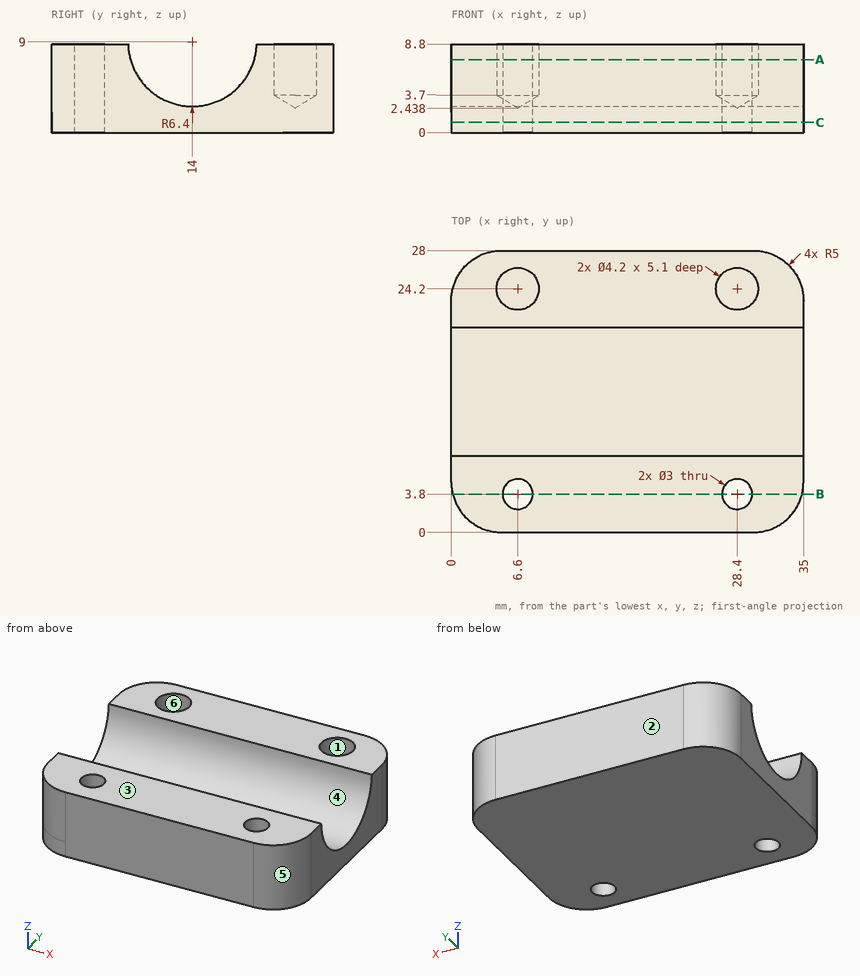
Geometry: see drawing. Coordinates: mm, zero at the bounding-box minimum. A direction names the side the tool comes from. Give positions to 0.01 mm unless a question says otherwise; leave off trailing zeros. Write each loop counter-clockwise with the first axis right and the second up, starting at its lowest first coordinate (ties: lowest second). Pieces come first, ordered by that corner, then holes. Notation, with made-up numbers: M -39,68 L 11,68 A20 cw 11,78 Z; hole C -38.5,-5 d5. An arc over 180 degrees is marked long. Return JSON: item names as keys, results as strings. Group by question number.
1) Cut plane A-A, the plane z = 7.25. Output: boundary loops of the cut face in (x, y), then the cut area to 3 significant figures.
2) Set-up query: the marked faces 1 and 2. Return all of +Z, -Z, +X, -X, +Y, -Y with unobstructed straight access to the full face (end or side cutting, diameter ignored); none if empty.
3) First-contact query: pin 1 Ø2.5 at (x, y) = (6.6, 3.8) entering from -Z; pin 2 Ø4 at (x, y) = (25.5, 13.5) entering from +Z; pin 3 Ø6 at (x, y) = (7.5, 24) entering from +Z; pin 4 Ø2.5 at (x, y) = (6.6, 24.2) entering from +Z. Flat tips, straight axial feed; report the tip coordinate or a pass-through.
4) Cut plane C-C, the plane z = 1. Output: boundary loops of the cut face in (x, y).
5) Cut plane B-B, the plane y = 3.8. Output: boundary loops of the cut face in (x, z), then the cut area to 3 significant figures.
6) Draft query along Y for the marked faces 3, 4, 5 and 6. Return one class per face: released by +Y, released by -Y, zero draft, split by the parting line, or undercut.
7) Ray query, L1, parallel to Y at x = 28.4, z = 6; L2, parallel to X at y = 24.2, z = 6.15; L3, parallel to Z at x = 3, y = 19 (1 decimal). Return the intervals inside material, ascending.
Data:
{
 "1": {"outline": "M 0,5 A5 ccw 5,0 L 30,0 A5 ccw 35,5 L 35,7.84 L 0,7.84 Z; M 0,20.16 L 35,20.16 L 35,23 A5 ccw 30,28 L 5,28 A5 ccw 0,23 Z; hole C 6.6,24.2 d4.2; hole C 6.6,3.8 d3; hole C 28.4,24.2 d4.2; hole C 28.4,3.8 d3", "area": "486 mm²"},
 "2": {"face 1": "+Z", "face 2": "+Z, -Z, +X, -X, +Y"},
 "3": {"pin 1": "passes through", "pin 2": "stops at z = 3.11", "pin 3": "stops at z = 8.8", "pin 4": "stops at z = 3.19"},
 "4": {"outline": "M 0,5 A5 ccw 5,0 L 30,0 A5 ccw 35,5 L 35,23 A5 ccw 30,28 L 5,28 A5 ccw 0,23 Z; hole C 6.6,3.8 d3; hole C 28.4,3.8 d3"},
 "5": {"outline": "M 0.15,0 L 5.1,0 L 5.1,8.8 L 0.15,8.8 Z; M 8.1,0 L 26.9,0 L 26.9,8.8 L 8.1,8.8 Z; M 29.9,0 L 34.85,0 L 34.85,8.8 L 29.9,8.8 Z", "area": "253 mm²"},
 "6": {"face 3": "zero draft", "face 4": "undercut", "face 5": "released by -Y", "face 6": "undercut"},
 "7": {"L1": "y = 0 to 2.3, 5.3 to 8.35, 19.65 to 22.1, 26.3 to 28", "L2": "x = 0.15 to 4.5, 8.7 to 26.3, 30.5 to 34.85", "L3": "z = 0 to 5"}
}
